For this review, take the finished solid that the model builds, in its own axes (mm). A direction names the side the tool comes from. Coordinates: 2 decimals unless noted, no trailing zeros. Loops run counter-clockwise (first coordinate to the right, second up) from the corner with the lowest first, then second, coordinate; pieces in that order, holes last. Notation, with made-up numbers: M 87,86.25 L 115,86.25 A8 ccw 115,94.25 Z; hole C 2.25,50.5 d9. An arc over 180 degrees is marked long. Put each result on its own line as item: value.
Autodesk Inventor part; units mm, degrees
ref_plane "YZ Plane" through (0, 0, 0) normal (1, 0, 0) x (0, 1, 0)
ref_plane "XZ Plane" through (0, 0, 0) normal (0, 1, 0) x (-1, 0, 0)
ref_plane "XY Plane" through (0, 0, 0) normal (0, 0, 1) x (1, 0, 0)
sketch "Sketch1" plane through (0, 0, 0) normal (0, 1, 0) x (-1, 0, 0)
  circle A0 centre (0, 0) radius 22.5
  dimension "d0" = 45
extrude "Extrusion1" add sketch "Sketch1" along normal blind 5
sketch "Sketch2" plane through (0, 5, 0) normal (0, 1, 0) x (1, 0, 0)
  line L0 (0, 0) -> (0, 8) construction
  line L1 (0, 0) -> (0, -8) construction
  circle A0 centre (0, 8) radius 1.9
  circle A1 centre (0, 0) radius 1.9
  circle A2 centre (0, -8) radius 1.9
  dimension "d3" = 8
  dimension "d4" = 8
  dimension "d5" = 3.8
  dimension "d6" = 3.8
  dimension "d7" = 3.8
extrude "Extrusion2" add sketch "Sketch2" along normal blind 10
sketch "Sketch7" plane through (0, 0, 0) normal (0, -1, 0) x (1, 0, 0)
  circle A0 centre (0, 0) radius 16.5 construction
  circle A1 centre (0, 16.5) radius 0.85
  circle A2 centre (16.5, 0) radius 0.85
  circle A3 centre (-16.5, 0) radius 0.85
  circle A4 centre (0, -16.5) radius 0.85
  dimension "d42" = 33
  dimension "d43" = 1.7
  dimension "d44" = 1.7
  dimension "d45" = 1.7
  dimension "d46" = 1.7
extrude "Extrusion6" cut sketch "Sketch7" against normal blind 5
sketch "Sketch8" plane through (0, 0, 0) normal (0, -1, 0) x (1, 0, 0)
  circle A0 centre (0, 0) radius 21
  dimension "d49" = 42
extrude "Extrusion7" cut sketch "Sketch8" against normal blind 1
sketch "Sketch9" plane through (0, 1, 0) normal (0, -1, 0) x (1, 0, 0)
  circle A0 centre (0, 0) radius 4.75
  line L0 (0, 0) -> (6, 0) construction
  line L1 (6, 0) -> (6, 6) construction
  line L2 (6, 6) -> (0, 6) construction
  line L3 (0, 6) -> (0, 0) construction
  line L4 (0, 0) -> (6, 6) construction
  line L5 (6, 6) -> (5.6464, 6.3536) construction
  line L6 (5.6464, 6.3536) -> (-5.6673, -4.9602)
  line L7 (-5.6673, -4.9602) -> (-4.9602, -5.6673)
  line L8 (-4.9602, -5.6673) -> (6.3536, 5.6464)
  line L9 (6.3536, 5.6464) -> (5.6464, 6.3536)
  dimension "d52" = 9.5
  dimension "d53" = 6
  dimension "d54" = 6
  dimension "d55" = 0.5
  dimension "d56" = 16
  dimension "d57" = 1
extrude "Extrusion8" cut sketch "Sketch9" against normal blind 1
properties part number "Motor Mount Fancy"
(1) Add section C-C (y = 11.25). Write out the cut boundary in (x, z), plus the area to 3 significant figures.
Determined:
outline: C 0,-8 d3.8; C 0,0 d3.8; C 0,8 d3.8
area: 34.0 mm^2
(2) Add section D-D (z = 16.5). Write out the cut boundary in (x, y).
Determined:
outline: M -15.3,0 L -12.99,0 L -12.99,1 L -0.85,1 L -0.85,5 L -15.3,5 Z; M 0.85,1 L 12.99,1 L 12.99,0 L 15.3,0 L 15.3,5 L 0.85,5 Z
(3) For pin 1 (6 mm diameter, centred on y = 3.5, z = 1.5, fed in from +X); pin 2 (3.5 mm diameter, centred on x = -2.5, z = -2.5, fed in from -Y); pin 3 (6 mm diameter, centred on x = 3, y = 4.5, fed in from -Z); pin 4 (2 mm diameter, centred on x = 0, z = 16.5, fed in from +Y), all flat-tipped, find the tip position at first contact; note any pin that passes through.
Determined:
pin 1: stops at x = 22.5
pin 2: stops at y = 1
pin 3: stops at z = -22.5
pin 4: stops at y = 5
(4) Tool access review of faces 4 (the cylindrical face through (-0.412, 9.93, 6.145)), 5 (the flat face through (0, 15, 0)), 6 (the flat face through (-4.667, 1.493, -3.96)): name each direction out of +Z, -Z, +X, -X, +Y, -Y from which nothing blocks a thin tool from reaching the whole face with its end or side.
Determined:
face 4: +Y
face 5: +Z, -Z, +X, -X, +Y
face 6: -Y
(5) Wall thickness on line 1 along Z through (x, y) = (-1, 13); line 2 along Y through (x, z) = (-1, -18); line 3 along Z through (x, y) = (-1.5, 12.25): over which ranges is each line inside the solid? List them lowest first. Write a range as [from, to].
Determined:
line 1: z = [-9.62, -6.38], [-1.62, 1.62], [6.38, 9.62]
line 2: y = [1, 5]
line 3: z = [-9.17, -6.83], [-1.17, 1.17], [6.83, 9.17]
(6) Add section A-A (x = 0). State how many separate pieces and enclosed holes the cut face has, plus the area to 3 significant figures.
Determined:
separate pieces: 3
enclosed holes: 0
area: 274 mm^2
(7) Add section B-B (z = 0). Write out the cut boundary in (x, y), plus the area to 3 significant figures.
Determined:
outline: M -22.5,0 L -21,0 L -21,1 L -17.35,1 L -17.35,5 L -22.5,5 Z; M -15.65,1 L -4.75,1 L -4.75,2 L 4.75,2 L 4.75,1 L 15.65,1 L 15.65,5 L 1.9,5 L 1.9,15 L -1.9,15 L -1.9,5 L -15.65,5 Z; M 17.35,1 L 21,1 L 21,0 L 22.5,0 L 22.5,5 L 17.35,5 Z
area: 198 mm^2
(8) Draft analysis for pull direction X (two halves, no side actions). For faces 1 (the cylindrical face through (-1.9, 9.93, 0.08)), 2 (the flat face through (-20, 0, 7)), 3 (the flat face through (-3.987, 1.493, -4.694)), state which applies: +X half, -X half, draft (parallel to the pull), parting line (faces both ways), or undercut.
Determined:
face 1: parting line
face 2: draft
face 3: undercut
